The listing builds one solid part. Answer for the finished solid, in the listing's coordinates (mm). A direction names the side the tool comes from. Round coordinates to 2 decimals unless told otherwise and drop trailing zeros. Loops run counter-clockwise (first coordinate to the right, second up) from the corner with the lowest first, then second, coordinate; pieces in that order, holes last. Notation, with made-up numbers: (-20, -22.5) -> (-13, -22.5) arc R37 cw to (-13, 14.5) -> close; hole circle Ø6 at (9.25, -25.75). An arc over 180 degrees is marked (long way). One line per question, with ' | ' between items.
from build123d import *

# Parameters (mm, degrees)
BOX_W     = 40
BOX_H     = 40
BOX_DEPTH = 3
FILLET_R  = 1


with BuildPart() as fillet_body:
    # Box → Box (new body)
    with BuildSketch(Plane.XY.offset(-3)):
        with Locations((20, 20)):
            Rectangle(BOX_W, BOX_H)
    extrude(amount=BOX_DEPTH)

    # Fillet
    fillet_edges = [fillet_body.edges().sort_by_distance(p)[0] for p in [
        (0, 0, -1.5),
        (0, 40, -1.5),
        (40, 0, -1.5),
        (40, 40, -1.5),
    ]]
    fillet(fillet_edges, radius=FILLET_R)


with BuildPart() as fillet_body_1:
    # Fillet placement: moved
    add(fillet_body.part.moved(Location((-20, -19, 0))))


with BuildPart() as cone001:
    # Cone001 → Cone001 (revolve)
    with BuildSketch(Plane.XZ):
        Polygon((0, 0), (15, 0), (3, 40), (0, 40), align=None)
    revolve(axis=Axis((0, 0, 0), (0, 0, 1)))


with BuildPart() as fusion:
    # Cone → Cone (revolve)
    with BuildSketch(Plane.XZ):
        Polygon((0, 0), (16, 0), (4, 40), (0, 40), align=None)
    revolve(axis=Axis((0, 0, 0), (0, 0, 1)))

    # Cut: cut Cone001
    add(cone001.part, mode=Mode.SUBTRACT)

    # Fusion: union Fillet body
    add(fillet_body_1.part)


solid = fusion.part
Q1. For a pull along X with two mould halves and no side action, classify faces 3 (the face through (0, 0, 0)), 4 (the face through (0, 21, -2)), 5 (the face through (7.233, 2.278, 24.724)), 6 (the face through (-6.811, -5.222, 24.724)) as pulls with the +X half, pulls with the -X half, needs draft (parallel to the pull), parting line crosses it, or undercut.
Numbers:
face 3: undercut | face 4: needs draft | face 5: undercut | face 6: parting line crosses it
Q2. Find the intervals of material crossed by line 1 (Z direction, x = 13, y = -15); line 2 (X direction, y = -3.5, z = 0.5); line 3 (X direction, y = 9, z = 9.5), in increasing order. Write a range as from..to.
Numbers:
line 1: -3..0 | line 2: -15.46..-14.43, 14.43..15.46 | line 3: -9.59..-8.16, 8.16..9.59
Q3. A cutting plane is placed at A-A on x = 0. Give the vertices of the cut face in (y, z).
Numbers:
outline: (-19, -3) -> (21, -3) -> (21, 0) -> (16, 0) -> (4, 40) -> (3, 40) -> (15, 0) -> (-15, 0) -> (-3, 40) -> (-4, 40) -> (-16, 0) -> (-19, 0) -> close
Q4. A cutting plane is placed at D-D on z = 24. Give the vertices of the cut face in (x, y).
Numbers:
outline: circle Ø17.6 at (0, 0); hole circle Ø15.6 at (0, 0)
Q5. A cutting plane is placed at C-C on y = 0. Give the vertices of the cut face in (x, z).
Numbers:
outline: (-20, -3) -> (20, -3) -> (20, 0) -> (16, 0) -> (4, 40) -> (3, 40) -> (15, 0) -> (-15, 0) -> (-3, 40) -> (-4, 40) -> (-16, 0) -> (-20, 0) -> close
Q6. For faces 1 (the face through (9, 15, 0)), 2 (the face through (0, -19, -2)), determine the directions among +Z, -Z, +X, -X, +Y, -Y from which every point of the face is accessible in a straight line to the end or side of a thin tool.
Numbers:
face 1: +Z | face 2: +Z, -Z, +X, -X, -Y
Q7. A cutting plane is placed at B-B on z = 2. Give the vertices of the cut face in (x, y).
Numbers:
outline: circle Ø30.8 at (0, 0); hole circle Ø28.8 at (0, 0)
Q8. Given pin 1 Ø12 at (y, z) = (-0.5, 24) entering from +X; pin 2 Ø2 at (y, z) = (15, 13.5) entering from +X; pin 3 Ø3 at (y, z) = (13.5, 9) entering from -X; pin 4 Ø6 at (x, z) = (-6.5, 35) entering from -Y, each flat-ended and moving along its own axis, determine where each tip first touches the part or whether it passes through.
Numbers:
pin 1: x = 10.6 | pin 2: through | pin 3: x = -5.9 | pin 4: y = -4.5
